```python
from build123d import *

# Parameters (mm, degrees)
SKETCH1_W           = 55
SKETCH1_H           = 90
BOSS_EXTRUDE1_DEPTH = 85
SHELL1_T            = -3
BOSS_EXTRUDE4_DEPTH = 87
SKETCH5_W           = 16
SKETCH5_H           = 72
CUT_EXTRUDE2_DEPTH  = 34
BOSS_EXTRUDE5_DEPTH = 52.4


with BuildPart() as part:
    # Sketch1 → Boss-Extrude1 (new body)
    with BuildSketch(Plane(origin=(0, 0, 0), x_dir=(1, 0, 0), z_dir=(0, 1, 0))):
        Rectangle(SKETCH1_W, SKETCH1_H)
    extrude(amount=BOSS_EXTRUDE1_DEPTH)

    # Shell1
    shell1_openings = [part.faces().sort_by_distance(p)[0] for p in [
        (0, 85, 0),
    ]]
    offset(amount=SHELL1_T, openings=shell1_openings, kind=Kind.INTERSECTION)

    # Sketch4 → Boss-Extrude4 (add)
    with BuildSketch(Plane.XY.offset(45)):
        Polygon((-24.5, 36), (6.5, 3), (-24.5, 3), align=None)
    extrude(amount=-BOSS_EXTRUDE4_DEPTH)

    # Sketch5 → Cut-Extrude2 (cut)
    with BuildSketch(Plane.ZY.offset(27.5)):
        Rectangle(SKETCH5_W, SKETCH5_H)
    extrude(amount=-CUT_EXTRUDE2_DEPTH, mode=Mode.SUBTRACT)

    # Sketch7 → Boss-Extrude5 (add)
    with BuildSketch(Plane(origin=(27.5, 0, 0), x_dir=(0, 0, -1), z_dir=(1, 0, 0))):
        Polygon((-42, 36), (-42, 3), (-8, 3), align=None)
        Polygon((8, 3), (42, 3), (42, 36), align=None)
    extrude(amount=-BOSS_EXTRUDE5_DEPTH)


solid = part.part
```
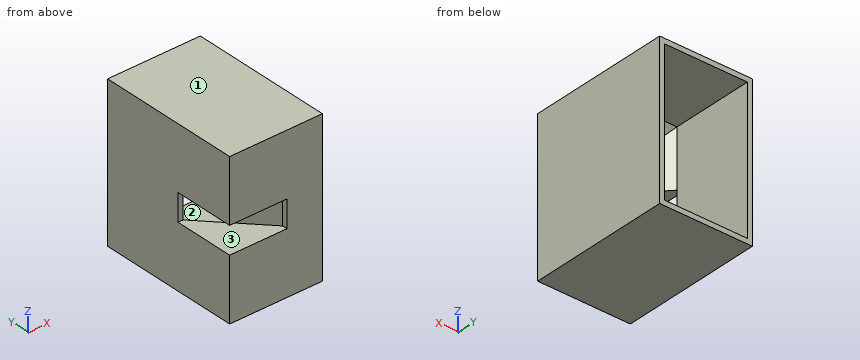
Can you work these out from the model? Positions are in its coordinate system, mm. Face numbers are marked on the shaded views. A direction names the side the tool comes from. Give positions to 0.01 mm unless a question says otherwise; leave off trailing zeros. Order: outer loops, then holes, each group sorted by start corner. A loop starts at its lowest first (then second) coordinate and runs counter-clockwise, first axis right, second up. Notation, with made-up numbers: (52, 73.25) - (110, 73.25) arc R24 cw to (110, 96.25) - close; hole circle Ø8 at (51.25, -17.5). An arc over 180 degrees is marked (long way). Use a Markdown table: item, result. Add a question column.
Q1. If we section it at D-D on x = 19.5: Write out the boundary of the cut face in (y, z), plus the area to 3 significant figures.
Q2. If we section it at B-B on y = 45: Write out the boundary of the cut face in (x, z), plus the area to 3 significant figures.
Q3. Please list where these lines run through material, in increasing order: line 1 along Z through (x, y) = (-13, 49.5); line 2 along X through (y, z) = (81, 31); line 3 along Z through (x, y) = (-9.5, 9.5).
Q4. On a 3-axis mill with a long thin cutter (end or side, diameter ignored), from which of +Z, -Z, +X, -X, +Y, -Y can I reach the whole of each face in a straight line? I mean the marked faces 1, 2 and 3. Say none if no direction works.
Q5. If we section it at A-A on x = -21: Write out the boundary of the cut face in (y, z), plus the area to 3 significant figures.
Q6. I'm going to push flat-ended pins straight in: pin 1 (8 mm diameter, centred on x = 4.5, z = -16, fed in from +Y); pin 2 (1.5 mm diameter, centred on x = -26, z = 3, fed in from -Y); pin 3 (10 mm diameter, centred on x = 5.5, z = 13, fed in from -Y); pin 4 (17.5 mm diameter, centred on x = 13, z = -3.5, fed in from +Y) (3 decimals). Where does each tip first touch, or does it pass through?
Q7. If we section it at C-C on z = -16.5: Write out the boundary of the cut face in (x, y), plus the area to 3 significant figures.
Answers follow:
| question | item | result |
|---|---|---|
| 1 | outline | (0, -45) - (85, -45) - (85, -42) - (36, -42) - (3, -8) - (3, 8) - (36, 42) - (85, 42) - (85, 45) - (0, 45) - close |
| 1 | area | 1,880 mm^2 |
| 2 | outline | (-27.5, -45) - (27.5, -45) - (27.5, 45) - (-27.5, 45) - close; hole (-24.5, -42) - (24.5, -42) - (24.5, 42) - (-24.5, 42) - close |
| 2 | area | 834 mm^2 |
| 3 | line 1 | z = -45 to -42, 42 to 45 |
| 3 | line 2 | x = -27.5 to -24.5, 24.5 to 27.5 |
| 3 | line 3 | z = -45 to -8, 8 to 45 |
| 4 | face 1 | +Z, +X, -X, +Y, -Y |
| 4 | face 2 | +Y |
| 4 | face 3 | -X, -Y |
| 5 | outline | (0, -45) - (85, -45) - (85, -42) - (36, -42) - (32.27, -38.16) - (32.27, -8) - (0, -8) - close; (0, 8) - (32.27, 8) - (32.27, 38.16) - (36, 42) - (85, 42) - (85, 45) - (0, 45) - close |
| 5 | area | 2,720 mm^2 |
| 6 | pin 1 | stops at y = 14.65 |
| 6 | pin 2 | stops at y = 36 |
| 6 | pin 3 | stops at y = 0 |
| 6 | pin 4 | stops at y = 7.125 |
| 7 | outline | (-27.5, 0) - (27.5, 0) - (27.5, 85) - (24.5, 85) - (24.5, 11.25) - (-1.25, 11.25) - (-24.5, 36) - (-24.5, 85) - (-27.5, 85) - close |
| 7 | area | 1,350 mm^2 |
